Part model, mm, in its own coordinate system. Face numbers are marked on the shaded views. Round coordinates to 2 decimals unless told otherwise and drop trailing zeros. Loops run counter-clockwise (first coordinate to the right, second up) from the corner with the lowest first, then second, coordinate; pieces in that order, holes last.
1) Band-saw the part on D-D, the plane x = 22.5. Write the cut outline in (y, z), then the cut area to 3 significant figures.
2) Probe line 1 (Z direction, x = 8, y = 2.4); line 2 (Z direction, x = 10, y = 3.45); line 3 (X direction, y = 2.35, z = 3). List the from-to ranges inside material, lowest first.
3) Band-saw the part on C-C, the plane y = 2.2. Write the cut outline in (x, z) (3 decimals), then the cut area to 3 significant figures.
4) Drop flat-ended pins along their axis: P1, Ø5.5, axis at x = -11, z = 0.5, coming from the +Y side; P2, Ø1.5, axis at y = 0.5, z = 20, coming from the -X side; P3, Ø5, axis at x = 6.71, z = -6.71, coming from the +Y side; P4, Ø1.5, axis at x = -1, y = 1.5, coming from the -Z side. Give the stop position or say it passes through.
5) Band-saw the part on A-A, the plane x = 0. Write the cut outline in (y, z), then the cut area to 3 significant figures.
6) Band-saw the part on B-B, the plane z = 0. Write the cut outline in (x, y), then the cut area to 3 significant figures.
7) Mould opens along Z. For the marked faces 1 and 2 say: +Z half, -Z half, draft (parallel to the pull), parting line (faces both ways), or undercut.
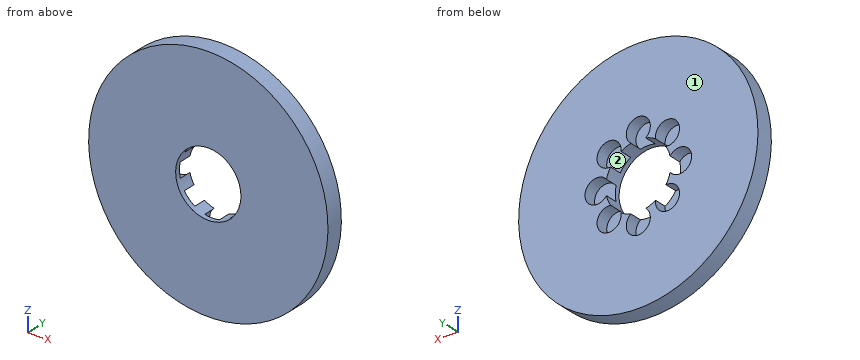
from build123d import *

# Parameters (mm, degrees)
SKETCH1_R           = 27.5
BOSS_EXTRUDE1_DEPTH = 4
SKETCH2_R           = 7.5
CUT_EXTRUDE1_DEPTH  = 40.096035605
SKETCH3_R           = 2.765377474
CUT_EXTRUDE2_DEPTH  = 2.872516
CIRPATTERN1_START   = 1.127483685
CIRPATTERN1_DEPTH   = 2.872516315


# Read off the part's stored shape, not the designer's step: CirPattern1
with BuildPart() as part:
    # Sketch1 → Boss-Extrude1 (new body)
    with BuildSketch(Plane(origin=(0, 0, 0), x_dir=(1, 0, 0), z_dir=(0, 1, 0))):
        with Locations(Location((0, 0, 0), (0, 0, 270))):
            Circle(SKETCH1_R)
    extrude(amount=BOSS_EXTRUDE1_DEPTH)

    # Sketch2 → Cut-Extrude1 (cut, through all)
    with BuildSketch(Plane(origin=(0, 0, 0), x_dir=(1, 0, 0), z_dir=(0, 1, 0))):
        with Locations(Location((0, 0, 0), (0, 0, 270))):
            Circle(SKETCH2_R)
    extrude(amount=CUT_EXTRUDE1_DEPTH, mode=Mode.SUBTRACT)

    # Sketch3 → Cut-Extrude2 (cut)
    with BuildSketch(Plane(origin=(0, 4, 0), x_dir=(1, 0, 0), z_dir=(0, 1, 0))):
        with Locations((-9.486828159, 0)):
            Circle(SKETCH3_R)
    extrude(amount=-CUT_EXTRUDE2_DEPTH, mode=Mode.SUBTRACT)

    # CirPattern1 outline → CirPattern1 (cut)
    with BuildSketch(Plane(origin=(0, 0, 0), x_dir=(1, 0, 0), z_dir=(0, 1, 0)).offset(CIRPATTERN1_START)):
        with BuildLine():
            ThreePointArc((-3.963970007, -6.36686279), (-5.303300859, -5.303300859), (-6.36686279, -3.963970007))
            ThreePointArc((-6.36686279, -3.963970007), (-8.663617688, -8.663617688), (-3.963970007, -6.36686279))
        make_face()
        with BuildLine():
            ThreePointArc((-3.963970007, 6.36686279), (-8.663617688, 8.663617688), (-6.36686279, 3.963970007))
            ThreePointArc((-6.36686279, 3.963970007), (-5.303300859, 5.303300859), (-3.963970007, 6.36686279))
        make_face()
        with BuildLine():
            ThreePointArc((1.699101781, -7.305001926), (0, -7.5), (-1.699101781, -7.305001926))
            ThreePointArc((-1.699101781, -7.305001926), (0, -12.252205633), (1.699101781, -7.305001926))
        make_face()
        with BuildLine():
            ThreePointArc((1.699101781, 7.305001926), (0, 12.252205633), (-1.699101781, 7.305001926))
            ThreePointArc((-1.699101781, 7.305001926), (0, 7.5), (1.699101781, 7.305001926))
        make_face()
        with BuildLine():
            ThreePointArc((6.36686279, -3.963970007), (5.303300859, -5.303300859), (3.963970007, -6.36686279))
            ThreePointArc((3.963970007, -6.36686279), (8.663617688, -8.663617688), (6.36686279, -3.963970007))
        make_face()
        with BuildLine():
            ThreePointArc((6.36686279, 3.963970007), (8.663617688, 8.663617688), (3.963970007, 6.36686279))
            ThreePointArc((3.963970007, 6.36686279), (5.303300859, 5.303300859), (6.36686279, 3.963970007))
        make_face()
        with BuildLine():
            ThreePointArc((7.305001926, 1.699101781), (7.5, 0), (7.305001926, -1.699101781))
            ThreePointArc((7.305001926, -1.699101781), (12.252205633, 0), (7.305001926, 1.699101781))
        make_face()
    extrude(amount=CIRPATTERN1_DEPTH, mode=Mode.SUBTRACT)


solid = part.part
Reported:
1. outline: (0, -15.81) - (4, -15.81) - (4, 15.81) - (0, 15.81) - close
1. area: 126 mm2
2. line 1: z = -26.31 to -9.15, -4.26 to -2.33, 2.33 to 4.26, 9.15 to 26.31
2. line 2: z = -25.62 to -2.72, 2.72 to 25.62
2. line 3: x = -27.34 to -6.87, 6.87 to 27.34
3. outline: circle Ø55 at (0, 0); hole (-7.305, -1.699) arc R7.5 ccw to (-6.367, -3.964) arc R2.765 ccw (long way) to (-3.964, -6.367) arc R7.5 ccw to (-1.699, -7.305) arc R2.765 ccw (long way) to (1.699, -7.305) arc R7.5 ccw to (3.964, -6.367) arc R2.765 ccw (long way) to (6.367, -3.964) arc R7.5 ccw to (7.305, -1.699) arc R2.765 ccw (long way) to (7.305, 1.699) arc R7.5 ccw to (6.367, 3.964) arc R2.765 ccw (long way) to (3.964, 6.367) arc R7.5 ccw to (1.699, 7.305) arc R2.765 ccw (long way) to (-1.699, 7.305) arc R7.5 ccw to (-3.964, 6.367) arc R2.765 ccw (long way) to (-6.367, 3.964) arc R7.5 ccw to (-7.305, 1.699) arc R2.765 ccw (long way) to start
3. area: 2,020 mm2
4. P1: stops at y = 4
4. P2: stops at x = -19.64
4. P3: stops at y = 1.13
4. P4: stops at z = -27.5
5. outline: (0, -27.5) - (4, -27.5) - (4, -12.25) - (1.13, -12.25) - (1.13, -7.5) - (0, -7.5) - close; (0, 7.5) - (1.13, 7.5) - (1.13, 12.25) - (4, 12.25) - (4, 27.5) - (0, 27.5) - close
5. area: 133 mm2
6. outline: (-27.5, 0) - (-7.5, 0) - (-7.5, 1.13) - (-12.25, 1.13) - (-12.25, 4) - (-27.5, 4) - close; (7.5, 0) - (27.5, 0) - (27.5, 4) - (12.25, 4) - (12.25, 1.13) - (7.5, 1.13) - close
6. area: 133 mm2
7. face 1: draft
7. face 2: undercut
